Here's how the part is built. I have some questions about the finished solid (model axes, mm). A direction names the side the tool comes from. Round coordinates to 2 decimals unless told otherwise and drop trailing zeros. Order: outer loops, then holes, each group sorted by start corner. A loop starts at its lowest first (then second) coordinate and runs counter-clockwise, first axis right, second up. Notation, with made-up numbers: M 85,57 L 120,57 A15 cw 120,72 Z; hole C -2,-12.5 d9. An arc over 180 degrees is marked long. Write item = value, one per line. Start each with the question number.
Item 1: I want a section at A-A, the plane z = -35.56. List the corners of the cut face in (x, y) for me.
Item 2: I want a section at B-B, the plane y = 9.5. State how many separate pieces and enclosed holes the cut face has, plus the area to 3 significant figures.
Item 3: We'd pull the mould along Z, two halves only. Please class faces 4 (the face through (35, 45, -27)), 5 (the face through (67.62, 22.18, -35.22)), 6 (the face through (67.3, 22.2, -3.8)): pulls with the +Z half, pulls with the -Z half, needs draft (parallel to the pull), parting line crosses it, or undercut.
Item 4: I'm going to push a flat-ended pin straight in: P1, Ø1.3, axis at y = 26.5, z = -1, coming from the +X side. Where does the tip first touch, or does it pass through?
Item 5: For faces 1 (the face through (67.62, 22.18, -7.28)), 2 (the face through (66.07, 22, -46)), 3 (the face through (66.07, 22, -1)), which set-ups out of +Z, -Z, +X, -X, +Y, -Y let a thin tool reach every point of the face, with its end or its side?
Item 6: Please list where these lines run through material, in increasing order: L1, parallel to Z at x = 33, y = 31; L2, parallel to Z at x = 29, y = 35.5; L3, parallel to X at y = 33.5, z = -36.
```python
from build123d import *

# Parameters (mm, degrees)
SALIENTE_EXTRUIR1_DEPTH = 45
DRILLS_R                = 1.5875
CORTAR_EXTRUIR1_DEPTH   = 98.843568471
PINOUT_R                = 0.254
CORTAR_EXTRUIR2_DEPTH   = 98.843568471


with BuildPart() as part:
    # Board → Saliente-Extruir1 (new body)
    with BuildSketch(Plane(origin=(0, 0, 0), x_dir=(1, 0, 0), z_dir=(0, 1, 0))):
        Polygon((68.55, 37.846), (68.55, 5.08), (66.07, 2.54), (66.07, 0), (0, 0), (0, 53.378473106), (64.505207648, 53.378473106), (66.07, 51.813680753), (66.07, 40.386), align=None)
    extrude(amount=SALIENTE_EXTRUIR1_DEPTH)

    # Drills → Cortar-Extruir1 (cut, through all)
    with BuildSketch(Plane(origin=(0, 0, 0), x_dir=(1, 0, 0), z_dir=(0, 1, 0))):
        with Locations(Location((15.27, 50.8, 0), (0, 0, 90))):
            Circle(DRILLS_R)
        with Locations(Location((66.07, 35.56, 0), (0, 0, 90))):
            Circle(DRILLS_R)
        with Locations(Location((66.07, 7.62, 0), (0, 0, 90))):
            Circle(DRILLS_R)
        with Locations(Location((13.970000009, 2.54, 0), (0, 0, 90))):
            Circle(DRILLS_R)
    extrude(amount=CORTAR_EXTRUIR1_DEPTH, mode=Mode.SUBTRACT)

    # Pinout → Cortar-Extruir2 (cut, through all)
    with BuildSketch(Plane(origin=(0, 0, 0), x_dir=(1, 0, 0), z_dir=(0, 1, 0))):
        with Locations(Location((63.50000008, 2.54, 0), (0, 0, 270))):
            Circle(PINOUT_R)
        with Locations(Location((60.96000008, 2.54, 0), (0, 0, 270))):
            Circle(PINOUT_R)
        with Locations(Location((58.42000008, 2.54, 0), (0, 0, 270))):
            Circle(PINOUT_R)
        with Locations(Location((55.88000008, 2.54, 0), (0, 0, 270))):
            Circle(PINOUT_R)
        with Locations(Location((53.34000008, 2.54, 0), (0, 0, 270))):
            Circle(PINOUT_R)
        with Locations(Location((50.80000008, 2.54, 0), (0, 0, 270))):
            Circle(PINOUT_R)
        with Locations(Location((45.72000008, 2.54, 0), (0, 0, 270))):
            Circle(PINOUT_R)
        with Locations(Location((43.18000008, 2.54, 0), (0, 0, 270))):
            Circle(PINOUT_R)
        with Locations(Location((40.64000008, 2.54, 0), (0, 0, 270))):
            Circle(PINOUT_R)
        with Locations(Location((38.10000008, 2.54, 0), (0, 0, 270))):
            Circle(PINOUT_R)
        with Locations(Location((35.56000008, 2.54, 0), (0, 0, 270))):
            Circle(PINOUT_R)
        with Locations(Location((33.02000008, 2.54, 0), (0, 0, 270))):
            Circle(PINOUT_R)
        with Locations(Location((30.48000008, 2.54, 0), (0, 0, 270))):
            Circle(PINOUT_R)
        with Locations(Location((27.94000008, 2.54, 0), (0, 0, 270))):
            Circle(PINOUT_R)
        with Locations(Location((63.50000008, 50.8, 0), (0, 0, 270))):
            Circle(PINOUT_R)
        with Locations(Location((60.96000008, 50.8, 0), (0, 0, 270))):
            Circle(PINOUT_R)
        with Locations(Location((58.42000008, 50.8, 0), (0, 0, 270))):
            Circle(PINOUT_R)
        with Locations(Location((55.88000008, 50.8, 0), (0, 0, 270))):
            Circle(PINOUT_R)
        with Locations(Location((53.34000008, 50.8, 0), (0, 0, 270))):
            Circle(PINOUT_R)
        with Locations(Location((50.80000008, 50.8, 0), (0, 0, 270))):
            Circle(PINOUT_R)
        with Locations(Location((48.26000008, 50.8, 0), (0, 0, 270))):
            Circle(PINOUT_R)
        with Locations(Location((45.72000008, 50.8, 0), (0, 0, 270))):
            Circle(PINOUT_R)
        with Locations(Location((41.68600002, 50.8, 0), (0, 0, 270))):
            Circle(PINOUT_R)
        with Locations(Location((39.14600002, 50.8, 0), (0, 0, 270))):
            Circle(PINOUT_R)
        with Locations(Location((36.60600002, 50.8, 0), (0, 0, 270))):
            Circle(PINOUT_R)
        with Locations(Location((34.06600002, 50.8, 0), (0, 0, 270))):
            Circle(PINOUT_R)
        with Locations(Location((31.52600002, 50.8, 0), (0, 0, 270))):
            Circle(PINOUT_R)
        with Locations(Location((28.98600002, 50.8, 0), (0, 0, 270))):
            Circle(PINOUT_R)
        with Locations(Location((26.44600002, 50.8, 0), (0, 0, 270))):
            Circle(PINOUT_R)
        with Locations(Location((23.90600002, 50.8, 0), (0, 0, 270))):
            Circle(PINOUT_R)
        with Locations(Location((21.36600002, 50.8, 0), (0, 0, 270))):
            Circle(PINOUT_R)
        with Locations(Location((18.82600002, 50.8, 0), (0, 0, 270))):
            Circle(PINOUT_R)
    extrude(amount=CORTAR_EXTRUIR2_DEPTH, mode=Mode.SUBTRACT)


solid = part.part
```
Filled in:
q1.outline = M 0,0 L 64.48,0 L 64.48,45 L 0,45 Z; M 67.66,0 L 68.55,0 L 68.55,45 L 67.66,45 Z
q2.separate_pieces = 1
q2.enclosed_holes = 36
q2.area = 3,570 mm^2
q3.face_4 = needs draft
q3.face_5 = undercut
q3.face_6 = pulls with the +Z half
q4.P1 = 66.07
q5.face_1 = +Y, -Y
q5.face_2 = -Z, +X, +Y, -Y
q5.face_3 = +Z, +X, +Y, -Y
q6.L1 = -53.38 to -2.79, -2.29 to 0
q6.L2 = -53.38 to -51.05, -50.55 to 0
q6.L3 = 0 to 64.54, 67.6 to 68.55
